Design review of the part built by this model. Coordinates are the model's own, in mm. A direction names the side the tool comes from. Coordinates: 2 decimals unless noted, no trailing zeros. Loops run counter-clockwise (first coordinate to the right, second up) from the corner with the lowest first, then second, coordinate; pieces in that order, holes last. Notation, with made-up numbers: (-20.75, 35) -> (-7.75, 35) arc R9 cw to (-7.75, 48) -> close; hole circle Ø9 at (75, -19). An arc over 180 degrees is marked (long way). Answer as a JSON object with one key per item and string values.
```python
from build123d import *

# Parameters (mm, degrees)
F2_SIZE  = 2.54
F3_R     = 7.430416
F4_DEPTH = 25.4


with BuildPart() as f1:
    # F0 (on Front) → F1 (revolve)
    with BuildSketch(Plane.XZ):
        Polygon((0, 62.504839), (0, 0), (82.007878, 0), (82.007878, 12.843461), (40.337984, 12.843461), (40.337984, 25.972329), (14.080239, 25.972329), (14.080239, 62.504839), align=None)
    revolve(axis=Axis((41.003939, 0, 0), (1, 0, 0)))

    # F2
    f2_edges = [f1.edges().sort_by_distance(p)[0] for p in [
        (82.007878, 0, -12.843461),
    ]]
    chamfer(f2_edges, length=F2_SIZE)

    # F3 (on face) → F4 (cut)
    with BuildSketch(Plane.YZ.offset(14.080239)):
        with Locations((0, 44.809405)):
            Circle(F3_R)
        with Locations((-38.806083, 22.404702)):
            Circle(F3_R)
        with Locations((-38.806083, -22.404702)):
            Circle(F3_R)
        with Locations((0, -44.809405)):
            Circle(F3_R)
        with Locations((38.806083, -22.404702)):
            Circle(F3_R)
        with Locations((38.806083, 22.404702)):
            Circle(F3_R)
    extrude(amount=-F4_DEPTH, mode=Mode.SUBTRACT)


solid = f1.part
```
1) For faces 1 (the cylindrical face through (7.14, -44.7, 17.88)), 2 (the cylindrical face through (59.63, 12.54, -2.78)), list the 3-axis set-ups (+Z, -Z, +X, -X, +Y, -Y) from which the entire face can be reached by the end or side of a thin tool; tool diameter is ignored.
Completed:
{"face 1": "+X, -X", "face 2": "+X"}
2) Add section D-D, the plane x = 10. Give the boundary of the cut face in (y, z).
Completed:
{"outline": "circle Ø125.01 at (0, 0); hole circle Ø14.86 at (-38.81, -22.4); hole circle Ø14.86 at (-38.81, 22.4); hole circle Ø14.86 at (0, -44.81); hole circle Ø14.86 at (0, 44.81); hole circle Ø14.86 at (38.81, -22.4); hole circle Ø14.86 at (38.81, 22.4)"}
3) Clearance check with flat-ended pins moving along their axes: pin 1 Ø1.5 at (y, z) = (19, 4.5) entering from +X; pin 2 Ø17 at (y, z) = (-38.81, 22.4) entering from +X; pin 3 Ø1 at (x, z) = (40.5, -6) entering from +Y. State where each tip first meets the part, or that it passes through.
Completed:
{"pin 1": "x = 40.34", "pin 2": "x = 14.08", "pin 3": "y = 25.38"}
4) Add section A-A, the plane y = 0. Give the boundary of the cut face in (x, z).
Completed:
{"outline": "(0, -62.5) -> (14.08, -62.5) -> (14.08, -52.24) -> (0, -52.24) -> close; (0, -37.38) -> (14.08, -37.38) -> (14.08, -25.97) -> (40.34, -25.97) -> (40.34, -12.84) -> (79.47, -12.84) -> (82.01, -10.3) -> (82.01, 10.3) -> (79.47, 12.84) -> (40.34, 12.84) -> (40.34, 25.97) -> (14.08, 25.97) -> (14.08, 37.38) -> (0, 37.38) -> close; (0, 52.24) -> (14.08, 52.24) -> (14.08, 62.5) -> (0, 62.5) -> close"}
5) Wall thickness on probe 1 along Z at (x, y) = (10.5, 0); probe 2 along Z at (x, y) = (4, -42.5); probe 3 along X at (y, z) = (48.5, 17.5): over which ranges is each line inside the solid? List them lowest first.
Completed:
{"probe 1": "-62.5 to -52.24, -37.38 to 37.38, 52.24 to 62.5", "probe 2": "-45.83 to -28.85, -15.96 to 15.96, 28.85 to 45.83", "probe 3": "0 to 14.08"}
6) The part is to be moulded in two halves that separate along Y. For faces 3 (the cylindrical face through (7.14, -46.23, -22.08)), 4 (the flat face through (40.338, 5, 12)), 5 (the cylindrical face through (7.139, -0.967, -37.442)), 6 (the cylindrical face through (6.942, -2.748, -62.444)), say which applies: pulls with the +Y half, pulls with the -Y half, needs draft (parallel to the pull), parting line crosses it, or undercut.
Completed:
{"face 3": "undercut", "face 4": "needs draft", "face 5": "undercut", "face 6": "parting line crosses it"}
7) Add section C-C, the plane z = 0. Give the boundary of the cut face in (x, y).
Completed:
{"outline": "(0, -62.5) -> (14.08, -62.5) -> (14.08, -25.97) -> (40.34, -25.97) -> (40.34, -12.84) -> (79.47, -12.84) -> (82.01, -10.3) -> (82.01, 10.3) -> (79.47, 12.84) -> (40.34, 12.84) -> (40.34, 25.97) -> (14.08, 25.97) -> (14.08, 62.5) -> (0, 62.5) -> close"}
8) Add section B-B, the plane z = 39. Give the boundary of the cut face in (x, y).
Completed:
{"outline": "(0, -48.85) -> (14.08, -48.85) -> (14.08, -4.63) -> (0, -4.63) -> close; (0, 4.63) -> (14.08, 4.63) -> (14.08, 48.85) -> (0, 48.85) -> close"}
